Autodesk Inventor part; units mm, degrees
ref_plane "YZ Plane" through (0, 0, 0) normal (1, 0, 0) x (0, 1, 0)
ref_plane "XZ Plane" through (0, 0, 0) normal (0, 1, 0) x (-1, 0, 0)
ref_plane "XY Plane" through (0, 0, 0) normal (0, 0, 1) x (1, 0, 0)
sketch "Эскиз1" plane through (0, 0, 0) normal (1, 0, 0) x (0, 1, 0)
  line L0 (0, 100) -> (0, -100)
  line L1 (0, -100) -> (30, -100)
  line L2 (30, -100) -> (30, 100)
  line L3 (30, 100) -> (0, 100)
  line L4 (-14, 0) -> (84, 0) construction
  line L5 (0, -140) -> (0, 140) construction
  line L6 (30, -100) -> (70, -100)
  line L7 (70, -100) -> (70, 100)
  line L8 (70, 100) -> (30, 100)
  line L9 (30, 100) -> (30, -100)
  point P0 (0, 0)
  point P1 (30, 100)
  dimension "d0" = 200
  dimension "d1" = 30
  dimension "d2" = 200
  dimension "d3" = 40
extrude "Выдавливание1" add sketch "Эскиз1" along normal mid plane 12
sketch "Эскиз2" plane through (6, 0, 0) normal (1, 0, 0) x (0, 0, -1)
  line L0 (-20, 13) -> (-40, 13)
  line L1 (-100, 0) -> (100, 0) construction
  line L2 (100, 0) -> (100, 70)
  line L3 (-40, 13) -> (-20, 13)
  line L4 (-20, 13) -> (-20, 3)
  line L5 (-20, 3) -> (-40, 3)
  line L6 (-40, 3) -> (-40, 13)
  line L7 (20, 13) -> (40, 13)
  line L8 (40, 13) -> (40, 3)
  line L9 (40, 3) -> (20, 3)
  line L10 (20, 3) -> (20, 13)
  point P0 (0, 0)
  point P1 (-85, 0)
  point P2 (57.0517, 0.6179)
  dimension "d26" = 10
  dimension "d27" = 20
  dimension "d28" = 3
  dimension "d29" = 20
  dimension "d31" = 20
  dimension "d34" = 3
  dimension "d35" = 10
  dimension "d36" = 20
extrude "Выдавливание2" cut sketch "Эскиз2" against normal blind 12
sketch "Эскиз3" plane through (-6, 0, 0) normal (1, 0, 0) x (0, 0, -1)
  line L0 (100, 0) -> (100, 70)
  line L1 (100, 0) -> (-100, 0)
  line L2 (-100, 0) -> (-100, 70)
  point P0 (0, 0)
  point P1 (-85, 15)
  point P2 (-85, 0)
  point P3 (-85, 15)
  point P4 (85, 15)
  point P5 (-100, 15)
  dimension "d17" = 15
  dimension "d53" = 15
  dimension "d54" = 15
hole "Отверстие1" at (-6, 15, -85) at (-6, 15, 85) direction (1, 0, 0) diameter 14 depth 4.1
sketch "Эскиз4" plane through (6, 0, 0) normal (1, 0, 0) x (0, 0, -1)
  line L0 (100, 70) -> (-100, 70)
  line L1 (-100, 70) -> (-100, 0)
  line L2 (90, 30) -> (-85, 30)
  line L3 (100, 0) -> (100, 70)
  line L4 (100, 0) -> (-100, 0)
  point P0 (0, 0)
  point P1 (95, 65)
  point P2 (95, 37)
  point P3 (-100, 15)
  point P4 (-85, 0)
  dimension "d37" = 5
  dimension "d40" = 5
  dimension "d51" = 5
  dimension "d52" = 37
hole "Отверстие2" at (6, 65, -95) at (6, 37, -95) direction (-1, 0, 0) diameter 3 depth 70
chamfer "Фаска1" distance 0.2 angle 45 4 edges at (6, 37, -93.5) (6, 65, -93.5) (-6, 37, -93.5) (-6, 65, -93.5)
sketch "Эскиз5" plane through (-6, 70, 100) normal (0, 1, 0) x (1, 0, 0)
  line L0 (0, 0) -> (0, 200)
  line L1 (0, 17.3205) -> (10, 0)
  line L2 (12, 0) -> (0, 0)
  line L3 (0, 0) -> (10, 0)
  line L4 (0, 0) -> (0, 17.3205)
  point P0 (6, 100)
  dimension "d55" = 60
  dimension "d56" = 10
extrude "Выдавливание3" cut sketch "Эскиз5" against normal blind 40
sketch "Эскиз6" plane through (-6, 70, -100) normal (0, 1, 0) x (1, 0, 0)
  line L0 (0, 0) -> (12, 0)
  line L1 (10, -200) -> (0, -200)
  line L2 (0, -182.6795) -> (0, 0)
  point P0 (6, -100)
  point P1 (6, -40)
  point P2 (6, -160)
  dimension "d60" = 40
  dimension "d61" = 40
  dimension "d62" = 6
  dimension "d63" = 6
hole "Отверстие3" at (0, 70, -60) at (0, 70, 60) direction (0, -1, 0) diameter 8.1 depth 80
properties part number "Стенка конвейера"
Verification items for the finished model (mm, model axes). A direction names the side the tool comes from. Give positions to 0.01 mm unless a question says otherwise; leave off trailing zeros. Loops run counter-clockwise (first coordinate to the right, second up) from the corner with the lowest first, then second, coordinate; pieces in that order, holes last. Notation, with made-up numbers: (44, 5) - (82, 5) arc R29 cw to (82, 34) - close; hole circle Ø5 at (75.5, -9.5). An arc over 180 degrees is marked (long way). Write item = value, one per line. Start each with the question number.
Q1. Cross-section at C-C, the plane y = 40.5. Enter the section's corners in (x, z).
Q2. Cross-section at B-B, the plane z = 60. Enter the section's corners in (x, y).
Q3. Cross-section at D-D, the plane z = -33.5. Enter the section's corners in (x, y), and give its area (3 significant figures).
Q4. Depth check by flat-ended pin: P1, Ø5, axis at x = 0, z = 60, coming from the +Y side; P2, Ø7, axis at y = 14, z = 88, coming from the -X side; P3, Ø3.5, axis at y = 65, z = -95, coming from the -X side. Enter the tip coordinate at first touch or a pass-through.
Q5. Thickness scan on line 1 (Y direction, x = -3.25, z = -95); line 2 (Y direction, x = -4, z = 36.5); line 3 (Y direction, x = -2.8, z = -85). Record the ranges inside material, lowest first.
Q6. Cross-section at A-A, the plane y = 6. Enter the section's corners in (x, z).
Q7. Tool access check on faces 4 (the face through (-4, 15, -92)), 5 (the face through (-3, 30, 95)), 6 (the face through (0, 8, 40)), 7 (the face through (6, 35, 1)). Record the directions out of +Z, -Z, +X, -X, +Y, -Y that give a thin tool (end or side, any length) a straight path to the whole face; none if there is none.
Q8. Mould release check, pull along Z, two halves, no side actions. Record for faces 1 (the face through (-6, 35, 1)), 2 (the face through (0, 35, -100)), 3 (the face through (0, 8, -20)): released by +Z, released by -Z, zero draft, split by the parting line, or undercut.
Answer key:
q1.outline = (-6, -100) - (6, -100) - (6, 100) - (4, 100) - (-6, 82.68) - close; hole circle Ø8.1 at (0, -60); hole circle Ø8.1 at (0, 60)
q2.outline = (-6, 0) - (-4.05, 0) - (-4.05, 70) - (-6, 70) - close; (4.05, 0) - (6, 0) - (6, 70) - (4.05, 70) - close
q3.outline = (-6, 0) - (6, 0) - (6, 3) - (-6, 3) - close; (-6, 13) - (6, 13) - (6, 70) - (-6, 70) - close
q3.area = 720 mm^2
q4.P1 = through
q4.P2 = -1.9
q4.P3 = -6
q5.line_1 = 0 to 35.5, 38.5 to 63.5, 66.5 to 70
q5.line_2 = 0 to 3, 13 to 70
q5.line_3 = 0 to 8, 22 to 70
q6.outline = (-6, -100) - (6, -100) - (6, -40) - (-6, -40) - close; (-6, -20) - (6, -20) - (6, 20) - (-6, 20) - close; (-6, 40) - (6, 40) - (6, 100) - (-6, 100) - close; hole circle Ø8.1 at (0, -60); hole circle Ø8.1 at (0, 60)
q7.face_4 = -X
q7.face_5 = +Z, -X, +Y
q7.face_6 = +X, -X
q7.face_7 = +Z, -Z, +X, +Y, -Y
q8.face_1 = zero draft
q8.face_2 = released by -Z
q8.face_3 = undercut
